Job drawing, mm, ordinate dimensions from the low corner. One solid piece. Round coordinates to 2 decimals unless told otherwise and drop trailing zeros. Loops run counter-clockwise (first coordinate to the right, second up) from the corner with the lowest first, then second, coordinate; pieces in that order, holes last. Notation, with made-up numbers: M 2.5,54 L 14.5,54 A26 cw 14.5,72 Z; hole C -22.5,-13 d1. An arc over 180 degrees is marked long. Use a Markdown table: item, result. Add a question column.
(1) Band-saw the part on C-C, the plane z = 12.5. Write the cut outline in (x, y).
(2) Band-saw the part on D-D, the plane z = 24.25. Write the cut outline in (x, y) (1 decimal).
(3) Band-saw the part on B-B, the plane x = 14.5. Write the cut outline in (y, z).
(4) Wall check: L1, parallel to Z at x = 15.5, y = 0.35 (1 decimal); L2, parallel to X at y = 2.05, z = 12 (1 decimal); L3, parallel to X at y = 1.5, z = 13 (1 decimal). Give the ranges that are in metal, low to high.
(5) Band-saw the part on A-A, the plane y = 0.65. Write the cut outline in (x, z) (1 decimal), and give its area (3 significant figures).
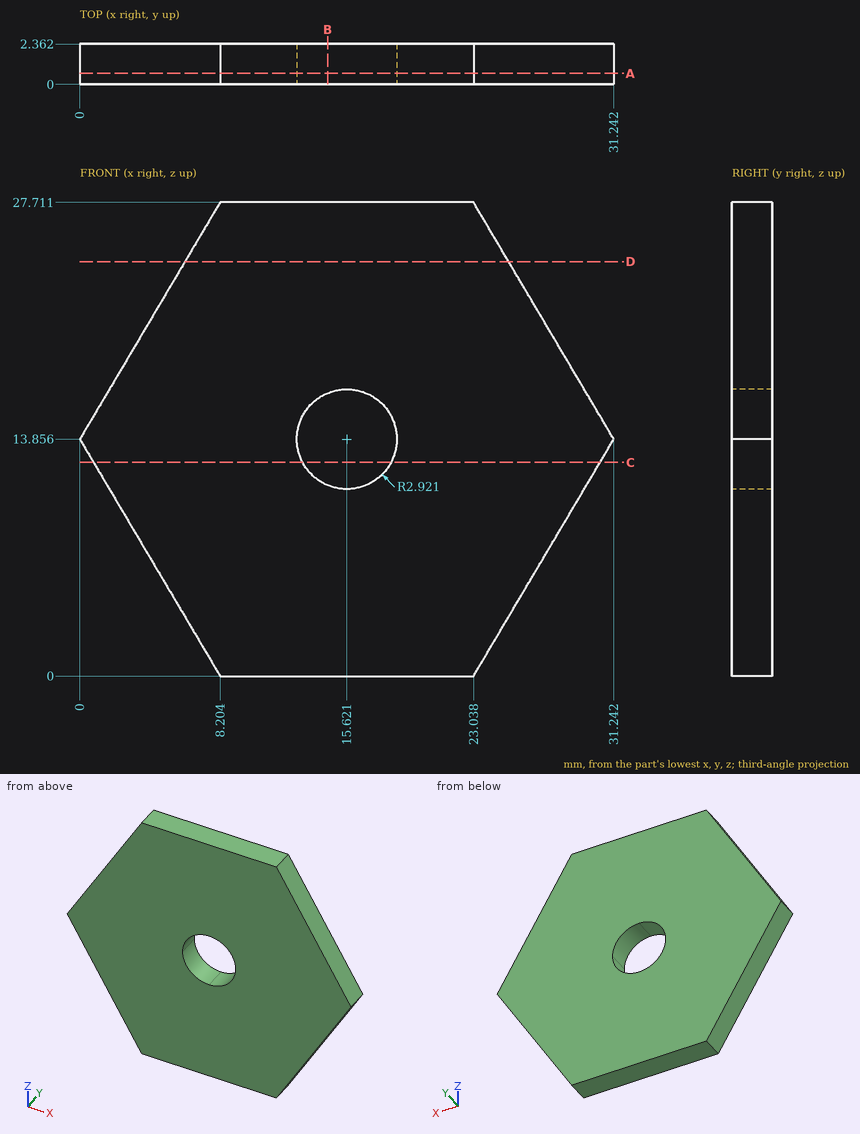
Return value:
| question | item | result |
|---|---|---|
| 1 | outline | M 0.8,0 L 13.03,0 L 13.03,2.36 L 0.8,2.36 Z; M 18.21,0 L 30.44,0 L 30.44,2.36 L 18.21,2.36 Z |
| 2 | outline | M 6.2,0 L 25.1,0 L 25.1,2.4 L 6.2,2.4 Z |
| 3 | outline | M 0,0 L 2.36,0 L 2.36,11.16 L 0,11.16 Z; M 0,16.55 L 2.36,16.55 L 2.36,27.71 L 0,27.71 Z |
| 4 | L1 | 0 to 10.9, 16.8 to 27.7 |
| 4 | L2 | 1.1 to 13.4, 17.9 to 30.1 |
| 4 | L3 | 0.5 to 12.8, 18.4 to 30.7 |
| 5 | outline | M 0,13.9 L 8.2,0 L 23,0 L 31.2,13.9 L 23,27.7 L 8.2,27.7 Z; hole C 15.6,13.9 d5.8 |
| 5 | area | 612 mm^2 |
